Work out the finished part from the listing and answer in its coordinate system (mm). A direction names the side the tool comes from. Coordinates: 2 decimals unless noted, no trailing zeros. Write each loop counter-clockwise with the first axis right and the second up, starting at its lowest first coordinate (ties: lowest second). Pieces come first, ordered by that corner, then holes. Notation, with made-up numbers: (-26.5, 1) - (24.5, 1) arc R20 ccw to (24.5, 22) - close; hole circle Ø1 at (86, 77). An arc over 180 degrees is marked (long way). Use one line per item in the form item = value. Start each with the question number.
Item 1: A cutting plane is placed at B-B (z = 11.5). Write down the section's boundary in (x, y) (3 decimals), then the cut area to 3 significant figures.
Item 2: Consider probe 1 along X at (y, z) = (-32, 11.5); probe 2 along Z at (x, y) = (30.5, 55); probe 3 along X at (y, z) = (21, 17). Determine where each line is inside the solid, lowest interval first.
Item 3: For faces 4 (the flat face through (0, 1, 25.908)), 5 (the flat face through (26.6, -55.6, 23.749)), 6 (the flat face through (-26.8, -58.5, 23.749)), determine the directions among +Z, -Z, +X, -X, +Y, -Y from which every point of the face is accessible in a straight line to the end or side of a thin tool.
Item 4: A cutting plane is placed at D-D (x = 9). Write down the section's boundary in (y, z) (3 decimals), then the cut area to 3 significant figures.
Item 5: A cutting plane is placed at A-A (y = 57.15). Give the number of separate pieces and of enclosed holes in the cut face, then the cut area to 3 significant figures.
Item 6: A cutting plane is placed at C-C (y = -7). Write down the section's boundary in (x, z) (3 decimals), then the cut area to 3 significant figures.
Item 7: Given pin 1 (1 mm diameter, centred on y = 9.5, z = 18.5, fed in from -X); pin 2 (1.7 mm diameter, centred on x = 25.5, z = 1.5, fed in from -Y); pin 3 (2.5 mm diameter, centred on x = 24, z = 24.5, fed in from +Y), each flat-ended and moving along its own axis, determine where each tip first touches the part or whether it passes through.
Item 8: Determine the mould class of faces 1 (the cylindrical face through (-28.706, -58.886, 24.844)), 2 (the cylindrical face through (34.67, 57.01, 24.84)), 3 (the cylindrical face through (-34.67, -57.01, 1.06)) for opening direction X: released by +X, released by -X, zero draft, split by the parting line, or undercut.
from build123d import *

# Parameters (mm, degrees)
F0_R     = 1.778
F1_DEPTH = 2.159
F2_W     = 43.18
F2_H     = 146.05
F3_DEPTH = 21.59
F4_R     = 1.778
F5_DEPTH = 2.159
F7_DEPTH = 146.051


# Not quite as in the source:
# - a pattern or mirror of a feature is missing from the dataset's text; its kind, count and spacing are read off the source's solid


with BuildPart() as f1:
    # F0 (on Top) → F1 (new body)
    with BuildSketch(Plane.XY):
        Polygon((21.59, 63.5), (21.59, 73.025), (-21.59, 73.025), (-21.59, 63.5), (-21.59, 50.8), (-21.59, -50.8), (-21.59, -63.5), (-21.59, -73.025), (21.59, -73.025), (21.59, -63.5), (21.59, -50.8), (21.59, 50.8), align=None)
        with BuildLine():
            Line((28.321, 63.5), (21.59, 63.5))
            Line((21.59, 63.5), (21.59, 50.8))
            Line((21.59, 50.8), (28.321, 50.8))
            ThreePointArc((28.321, 50.8), (34.671, 57.15), (28.321, 63.5))
        make_face()
        with Locations((28.321, 57.15)):
            Circle(F0_R, mode=Mode.SUBTRACT)
        with BuildLine():
            Line((-21.59, 50.8), (-21.59, 63.5))
            Line((-21.59, 63.5), (-28.321, 63.5))
            ThreePointArc((-28.321, 63.5), (-34.671, 57.15), (-28.321, 50.8))
            Line((-28.321, 50.8), (-21.59, 50.8))
        make_face()
        with Locations((-28.321, 57.15)):
            Circle(F0_R, mode=Mode.SUBTRACT)
        with BuildLine():
            Line((28.321, -50.8), (21.59, -50.8))
            Line((21.59, -50.8), (21.59, -63.5))
            Line((21.59, -63.5), (28.321, -63.5))
            ThreePointArc((28.321, -63.5), (34.671, -57.15), (28.321, -50.8))
        make_face()
        with Locations((28.321, -57.15)):
            Circle(F0_R, mode=Mode.SUBTRACT)
        with BuildLine():
            Line((-21.59, -63.5), (-21.59, -50.8))
            Line((-21.59, -50.8), (-28.321, -50.8))
            ThreePointArc((-28.321, -50.8), (-34.671, -57.15), (-28.321, -63.5))
            Line((-28.321, -63.5), (-21.59, -63.5))
        make_face()
        with Locations((-28.321, -57.15)):
            Circle(F0_R, mode=Mode.SUBTRACT)
    extrude(amount=F1_DEPTH)


with BuildPart() as f1_copies_1:
    # F1_copies: instance of F1
    add(f1.part.mirror(Plane.XY.offset(12.954)))


with BuildPart() as f1_1:
    add(f1.part)

    add(f1_copies_1.part)  # F3 merges F1_copies_1
    # F2 (on face) → F3 (join)
    with BuildSketch(Plane.XY.offset(2.159)):
        Rectangle(F2_W, F2_H)
    extrude(amount=F3_DEPTH)

    # F4 (on face) → F5 (join)
    with BuildSketch(Plane.XY):
        Polygon((21.59, 63.5), (21.59, 73.025), (-21.59, 73.025), (-21.59, 63.5), (-21.59, 50.8), (-21.59, -50.8), (-21.59, -63.5), (-21.59, -73.025), (21.59, -73.025), (21.59, -63.5), (21.59, -50.8), (21.59, 50.8), align=None)
        with BuildLine():
            Line((28.321, 63.5), (21.59, 63.5))
            Line((21.59, 63.5), (21.59, 50.8))
            Line((21.59, 50.8), (28.321, 50.8))
            ThreePointArc((28.321, 50.8), (34.671, 57.15), (28.321, 63.5))
        make_face()
        with Locations((28.321, 57.15)):
            Circle(F4_R, mode=Mode.SUBTRACT)
        with BuildLine():
            Line((-21.59, 50.8), (-21.59, 63.5))
            Line((-21.59, 63.5), (-28.321, 63.5))
            ThreePointArc((-28.321, 63.5), (-34.671, 57.15), (-28.321, 50.8))
            Line((-28.321, 50.8), (-21.59, 50.8))
        make_face()
        with Locations((-28.321, 57.15)):
            Circle(F4_R, mode=Mode.SUBTRACT)
        with BuildLine():
            Line((28.321, -50.8), (21.59, -50.8))
            Line((21.59, -50.8), (21.59, -63.5))
            Line((21.59, -63.5), (28.321, -63.5))
            ThreePointArc((28.321, -63.5), (34.671, -57.15), (28.321, -50.8))
        make_face()
        with Locations((28.321, -57.15)):
            Circle(F4_R, mode=Mode.SUBTRACT)
        with BuildLine():
            Line((-21.59, -63.5), (-21.59, -50.8))
            Line((-21.59, -50.8), (-28.321, -50.8))
            ThreePointArc((-28.321, -50.8), (-34.671, -57.15), (-28.321, -63.5))
            Line((-28.321, -63.5), (-21.59, -63.5))
        make_face()
        with Locations((-28.321, -57.15)):
            Circle(F4_R, mode=Mode.SUBTRACT)
    extrude(amount=F5_DEPTH)

    # F6 (on face) → F7 (cut, through all)
    with BuildSketch(Plane.XZ.offset(73.025)):
        with BuildLine():
            Line((-0.635, 9.9229806335), (-0.635, 15.9850193665))
            ThreePointArc((-0.635, 15.9850193665), (-18.7198, 12.954), (-0.635, 9.9229806335))
        make_face()
        with BuildLine():
            ThreePointArc((-0.635, 9.9229806335), (-0.2548795436, 11.4173524802), (-0.127, 12.954))
            ThreePointArc((-0.127, 12.954), (-0.2548795436, 14.4906475198), (-0.635, 15.9850193665))
            Line((-0.635, 15.9850193665), (-0.635, 9.9229806335))
        make_face()
        with BuildLine():
            Line((0.635, 9.9229806335), (0.635, 15.9850193665))
            ThreePointArc((0.635, 15.9850193665), (0.127, 12.954), (0.635, 9.9229806335))
        make_face()
        with BuildLine():
            ThreePointArc((18.7198, 12.954), (10.9600475198, 22.1225204564), (0.635, 15.9850193665))
            Line((0.635, 15.9850193665), (0.635, 9.9229806335))
            ThreePointArc((0.635, 9.9229806335), (10.9600475198, 3.7854795436), (18.7198, 12.954))
        make_face()
    extrude(amount=-F7_DEPTH, mode=Mode.SUBTRACT)


solid = f1_1.part
Answer:
q1.outline = (-21.59, -73.025) - (-18.605, -73.025) - (-18.605, 73.025) - (-21.59, 73.025) - close; (-0.241, -73.025) - (0.241, -73.025) - (0.241, 73.025) - (-0.241, 73.025) - close; (18.605, -73.025) - (21.59, -73.025) - (21.59, 73.025) - (18.605, 73.025) - close
q1.area = 942 mm²
q2.probe_1 = -21.59 to -18.61, -0.24 to 0.24, 18.61 to 21.59
q2.probe_2 = 0 to 2.16, 23.75 to 25.91
q2.probe_3 = -21.59 to -17.79, -1.05 to 1.05, 17.79 to 21.59
q3.face_4 = +Z, +X, -X, +Y, -Y
q3.face_5 = +X, +Y, -Y
q3.face_6 = -X, +Y, -Y
q4.outline = (-73.025, 0) - (73.025, 0) - (73.025, 3.667) - (-73.025, 3.667) - close; (-73.025, 22.241) - (73.025, 22.241) - (73.025, 25.908) - (-73.025, 25.908) - close
q4.area = 1,070 mm²
q5.separate_pieces = 5
q5.enclosed_holes = 2
q5.area = 658 mm²
q6.outline = (-21.59, 0) - (21.59, 0) - (21.59, 25.908) - (-21.59, 25.908) - close; hole circle Ø18.593 at (-9.423, 12.954); hole circle Ø18.593 at (9.423, 12.954)
q6.area = 576 mm²
q7.pin_1 = -21.59
q7.pin_2 = -63.5
q7.pin_3 = 63.5
q8.face_1 = undercut
q8.face_2 = released by +X
q8.face_3 = released by -X
